Geometry check sheet. Reference: the model listing, model coordinates, mm. A direction names the side the tool comes from. Round coordinates to 2 decimals unless told otherwise and drop trailing zeros. Order: outer loops, then holes, each group sorted by start corner. A loop starts at its lowest first (then second) coordinate and runs counter-clockwise, first axis right, second up.
(1) Cross-section at C-C on y = -9.25. Enter the section's corners in (x, z).
(2) Draft check along Z on faces 1 (the face through (19.697, -13, -24)), 2 (the face through (13.28, -12.88, 34.32)), 3 (the face through (1.68, -12.52, 56.31)). Enter one of: pulls with the +Z half, pulls with the -Z half, needs draft (parallel to the pull), parting line crosses it, or undercut.
(3) Gauge pin test, flat ends, axial feed: P1, Ø7.5, axis at y = -8, z = -20.5, coming from the -X side; P2, Ø12.5, axis at y = -18, z = -28.5, coming from the +X side; P3, Ø4, axis at x = 28, y = -3, coming from the +Z side. Record the tip position at first contact, or that the pin passes through.
(4) Cross-section at B-B on x = -18. Enter the section's corners in (y, z), and give its area (3 significant figures).
(5) Thickness scan on L1, parallel to X at y = -4.5, z = -15.5; L2, parallel to X at y = -12.75, z = 33; L3, parallel to Z at x = 0.5, y = -21. Record the ranges inside material, lowest first.
(6) Cross-section at A-A on z = -28. Enter the section's corners in (x, y).
(7) Cross-section at D-D on z = 26. Enter the section's corners in (x, y), and give its area (3 significant figures).
(8) Set-up check for faces 4 (the face through (14, -13, -36.493)), 5 (the face through (7.951, -13, -24)), 6 (the face through (-20.003, -13, -23)): record each of +Z, -Z, +X, -X, +Y, -Y from which the full face is reachable in a straight line by a thin tool's end or side.
from build123d import *

# Parameters (mm, degrees)
F1_DEPTH = 25.4
F2_W     = 1.488530077
F2_H     = 25.6520612165
F2_W_2   = 0.9923540056
F2_H_2   = 25.346679613
F3_DEPTH = 25.4
F4_R     = 7.6893132266
F4_R_2   = 7.0502845775
F5_DEPTH = 25.4


with BuildPart() as f1:
    # F0 (on Front) → F1 (new body)
    with BuildSketch(Plane.XZ):
        with BuildLine():
            Line((19.6971185505, -36.4931114018), (19.6971185505, -11.1464317888))
            ThreePointArc((19.6971185505, -11.1464317888), (0.3652750896, 56.3419043865), (-20.0025010854, -10.8410501853))
            Line((-20.0025010854, -10.8410501853), (-20.0025010854, -36.4931114018))
            Line((-20.0025010854, -36.4931114018), (-7.4818506837, -36.4931114018))
            Line((-7.4818506837, -36.4931114018), (6.8710884079, -36.4931114018))
            Line((6.8710884079, -36.4931114018), (19.6971185505, -36.4931114018))
        make_face()
    extrude(amount=F1_DEPTH)

    # F2 (on face) → F3 (cut)
    with BuildSketch(Plane.XZ.offset(25.4)):
        with Locations((-11.6479513235, -23.6670807935)):
            Rectangle(F2_W, F2_H)
        with Locations((8.4472019225, -23.8197715953)):
            Rectangle(F2_W_2, F2_H_2)
    extrude(amount=-F3_DEPTH, mode=Mode.SUBTRACT)

    # F4 (on face) → F5 (cut)
    with BuildSketch(Plane.XZ.offset(25.4)):
        with Locations((-15.4217751697, 27.3316595703)):
            Circle(F4_R)
        with Locations((14.2002468929, 27.3316595703)):
            Circle(F4_R_2)
    extrude(amount=-F5_DEPTH, mode=Mode.SUBTRACT)


solid = f1.part
Found:
1. outline: (-20, -36.49) - (-12.39, -36.49) - (-12.39, -10.84) - (-10.9, -10.84) - (-10.9, -36.49) - (7.95, -36.49) - (7.95, -11.15) - (8.94, -11.15) - (8.94, -36.49) - (19.7, -36.49) - (19.7, -11.15) arc R36.59 ccw (long way) to (-20, -10.84) - close; hole circle Ø15.38 at (-15.42, 27.33); hole circle Ø14.1 at (14.2, 27.33)
2. face 1: needs draft
2. face 2: undercut
2. face 3: parting line crosses it
3. P1: stops at x = -20
3. P2: stops at x = 19.7
3. P3: stops at z = 45.58
4. outline: (-25.4, -36.49) - (0, -36.49) - (0, 20.09) - (-25.4, 20.09) - close; (-25.4, 34.58) - (0, 34.58) - (0, 51.56) - (-25.4, 51.56) - close
4. area: 1,870 mm2
5. L1: x = -20 to -12.39, -10.9 to 7.95, 8.94 to 19.7
5. L2: x = -34.03 to -20.62, -10.23 to 10.01, 18.39 to 34.19
5. L3: z = -36.49 to 56.34
6. outline: (-20, -25.4) - (-12.39, -25.4) - (-12.39, 0) - (-20, 0) - close; (-10.9, -25.4) - (7.95, -25.4) - (7.95, 0) - (-10.9, 0) - close; (8.94, -25.4) - (19.7, -25.4) - (19.7, 0) - (8.94, 0) - close
7. outline: (-35.97, -25.4) - (-22.99, -25.4) - (-22.99, 0) - (-35.97, 0) - close; (-7.85, -25.4) - (7.28, -25.4) - (7.28, 0) - (-7.85, 0) - close; (21.12, -25.4) - (36.14, -25.4) - (36.14, 0) - (21.12, 0) - close
7. area: 1,100 mm2
8. face 4: -Z, +X, -X, +Y, -Y
8. face 5: -Z, +Y, -Y
8. face 6: -Z, -X, +Y, -Y
